```python
from build123d import *

# Parameters (mm, degrees)
SKETCH_1_W          = 60
SKETCH_1_H          = 60
EXTRUDE_1_DEPTH     = 124.5
SKETCH_2_R          = 25
EXTRUDE_2_DEPTH     = 3
SKETCH_3_R          = 7
EXTRUDE_3_DEPTH     = 27
SKETCH_4_R          = 2.75
CUT_EXTRUDE_1_DEPTH = 151.666021385
CUT_EXTRUDE_2_DEPTH = 118.5
FILLET_1_R          = 2


with BuildPart() as part:
    # 草图1 → 拉伸1 (new body)
    with BuildSketch(Plane.XY):
        with Locations((30, -30)):
            Rectangle(SKETCH_1_W, SKETCH_1_H)
    extrude(amount=EXTRUDE_1_DEPTH)

    # 草图2 → 拉伸2 (add)
    with BuildSketch(Plane.XY.offset(124.5)):
        with Locations((30, -30)):
            Circle(SKETCH_2_R)
    extrude(amount=EXTRUDE_2_DEPTH)

    # 草图3 → 拉伸3 (add)
    with BuildSketch(Plane.XY.offset(127.5)):
        with Locations((30, -30)):
            Circle(SKETCH_3_R)
    extrude(amount=EXTRUDE_3_DEPTH)

    # 草图4 → 切除-拉伸1 (cut, through all)
    with BuildSketch(Plane.XY.offset(124.5)):
        with Locations((54.748737342, -5.251262658)):
            Circle(SKETCH_4_R)
        with Locations((54.748737342, -54.748737342)):
            Circle(SKETCH_4_R)
        with Locations((5.251262658, -54.748737342)):
            Circle(SKETCH_4_R)
        with Locations((5.251262658, -5.251262658)):
            Circle(SKETCH_4_R)
    extrude(amount=-CUT_EXTRUDE_1_DEPTH, mode=Mode.SUBTRACT)

    # 草图5 → 切除-拉伸2 (cut)
    with BuildSketch(Plane(origin=(0, 0, 0), x_dir=(-1, 0, 0), z_dir=(0, 0, -1))):
        with BuildLine():
            Line((-10.502525317, -5.251262658), (-10.502525317, 0))
            Line((-10.502525317, 0), (0, 0))
            Line((0, 0), (0, -10.502525317))
            Line((0, -10.502525317), (-5.251262658, -10.502525317))
            ThreePointArc((-5.251262658, -10.502525317), (-8.964466094, -8.964466094), (-10.502525317, -5.251262658))
        make_face()
        with BuildLine():
            Line((-49.497474683, -54.748737342), (-49.497474683, -60))
            Line((-49.497474683, -60), (-60, -60))
            Line((-60, -60), (-60, -49.497474683))
            Line((-60, -49.497474683), (-54.748737342, -49.497474683))
            ThreePointArc((-54.748737342, -49.497474683), (-51.035533906, -51.035533906), (-49.497474683, -54.748737342))
        make_face()
        with BuildLine():
            Line((-60, 0), (-49.497474683, 0))
            Line((-49.497474683, 0), (-49.497474683, -5.251262658))
            ThreePointArc((-49.497474683, -5.251262658), (-51.035533906, -8.964466094), (-54.748737342, -10.502525317))
            Line((-54.748737342, -10.502525317), (-60, -10.502525317))
            Line((-60, -10.502525317), (-60, 0))
        make_face()
        with BuildLine():
            Line((0, -60), (-10.502525317, -60))
            Line((-10.502525317, -60), (-10.502525317, -54.748737342))
            ThreePointArc((-10.502525317, -54.748737342), (-8.964466094, -51.035533906), (-5.251262658, -49.497474683))
            Line((-5.251262658, -49.497474683), (0, -49.497474683))
            Line((0, -49.497474683), (0, -60))
        make_face()
    extrude(amount=-CUT_EXTRUDE_2_DEPTH, mode=Mode.SUBTRACT)

    # 圆角1
    fillet_1_edges = [part.edges().sort_by_distance(p)[0] for p in [
        (10.502525317, 0, 59.25),
        (0, -10.502525317, 59.25),
        (49.497474683, -60, 59.25),
        (60, -49.497474683, 59.25),
        (60, -10.502525317, 59.25),
        (49.497474683, 0, 59.25),
        (0, -49.497474683, 59.25),
        (10.502525317, -60, 59.25),
    ]]
    fillet(fillet_1_edges, radius=FILLET_1_R)


solid = part.part
```
The listing builds one solid part. Answer for the finished solid, in the listing's coordinates (mm). A direction names the side the tool comes from. Round coordinates to 2 decimals unless told otherwise and drop trailing zeros. Loops run counter-clockwise (first coordinate to the right, second up) from the corner with the lowest first, then second, coordinate; pieces in that order, holes last. Notation, with made-up numbers: (24, -14) -> (39, -14) arc R17 cw to (39, 4) -> close; hole circle Ø10 at (-15, 9). An arc over 180 degrees is marked (long way). Use one line per item in the form item = value.
1. The part is cut by section D-D on x = 15.5. Determine the outline of the cut face in (y, z).
Answer key:
outline = (-60, 0) -> (0, 0) -> (0, 124.5) -> (-9.63, 124.5) -> (-9.63, 127.5) -> (-50.37, 127.5) -> (-50.37, 124.5) -> (-60, 124.5) -> close
2. The part is cut by section C-C on x = 30. Determine the outline of the cut face in (y, z).
Answer key:
outline = (-60, 0) -> (0, 0) -> (0, 124.5) -> (-5, 124.5) -> (-5, 127.5) -> (-23, 127.5) -> (-23, 154.5) -> (-37, 154.5) -> (-37, 127.5) -> (-55, 127.5) -> (-55, 124.5) -> (-60, 124.5) -> close
3. A tool of negligible diameter and unlimited length cuts with its end or side. For faces 1 (the flat face through (56, -10.503, 58)), 2 (the flat face through (4, -49.497, 58)), 3 (the cylindrical face through (10, -45, 126)), 4 (the flat face through (4, -10.503, 58)), from which of +Z, -Z, +X, -X, +Y, -Y can it reach the whole face along a straight path? Write none if from no direction.
Answer key:
face_1 = -Z, +X, +Y
face_2 = -Z, -X, -Y
face_3 = +Z
face_4 = -Z, -X, +Y
4. The part is cut by section B-B on y = -30. Determine the outline of the cut face in (x, z), and give its area (3 significant figures).
Answer key:
outline = (0, 0) -> (60, 0) -> (60, 124.5) -> (55, 124.5) -> (55, 127.5) -> (37, 127.5) -> (37, 154.5) -> (23, 154.5) -> (23, 127.5) -> (5, 127.5) -> (5, 124.5) -> (0, 124.5) -> close
area = 8,000 mm²
5. For a pull along Y with two mould halves and no side action, classify faces 5 (the cylindrical face through (52.566, -56.422, 121.542)), 6 (the flat face through (3, -30, 124.5)), 7 (the cylindrical face through (8.92, -9.01, 58.42)) as released by +Y, released by -Y, zero draft, split by the parting line, or undercut.
Answer key:
face_5 = undercut
face_6 = zero draft
face_7 = released by +Y
6. Find the intervals of material crossed by probe 1 along Z at (x, y) = (56.5, -23); probe 2 along Z at (x, y) = (13.5, -29); probe 3 along X at (y, z) = (-29.5, 140.5), in increasing order. Write a range as [from, to].
Answer key:
probe_1 = [0, 124.5]
probe_2 = [0, 127.5]
probe_3 = [23.02, 36.98]
7. The part is cut by section A-A on z = 60.5. Determine the outline of the cut face in (x, y).
Answer key:
outline = (0, -47.5) arc R2 ccw to (2, -49.5) -> (5.25, -49.5) arc R5.25 cw to (10.5, -54.75) -> (10.5, -58) arc R2 ccw to (12.5, -60) -> (47.5, -60) arc R2 ccw to (49.5, -58) -> (49.5, -54.75) arc R5.25 cw to (54.75, -49.5) -> (58, -49.5) arc R2 ccw to (60, -47.5) -> (60, -12.5) arc R2 ccw to (58, -10.5) -> (54.75, -10.5) arc R5.25 cw to (49.5, -5.25) -> (49.5, -2) arc R2 ccw to (47.5, 0) -> (12.5, 0) arc R2 ccw to (10.5, -2) -> (10.5, -5.25) arc R5.25 cw to (5.25, -10.5) -> (2, -10.5) arc R2 ccw to (0, -12.5) -> close
8. Flat-ended cylindrical pins translate along their axes: pin 1 Ø3.5 at (x, y) = (5.25, -54.75) entering from +Z; pin 2 Ø1 at (x, z) = (3.5, 67) entering from +Y; pin 3 Ø1 at (x, z) = (4, 62) entering from -Y; pin 4 Ø2 at (x, y) = (40.5, -26) entering from +Z. Find the tip coordinate at first contact, or state that the pin passes through.
Answer key:
pin_1 = through
pin_2 = -10.5
pin_3 = -49.5
pin_4 = 127.5
